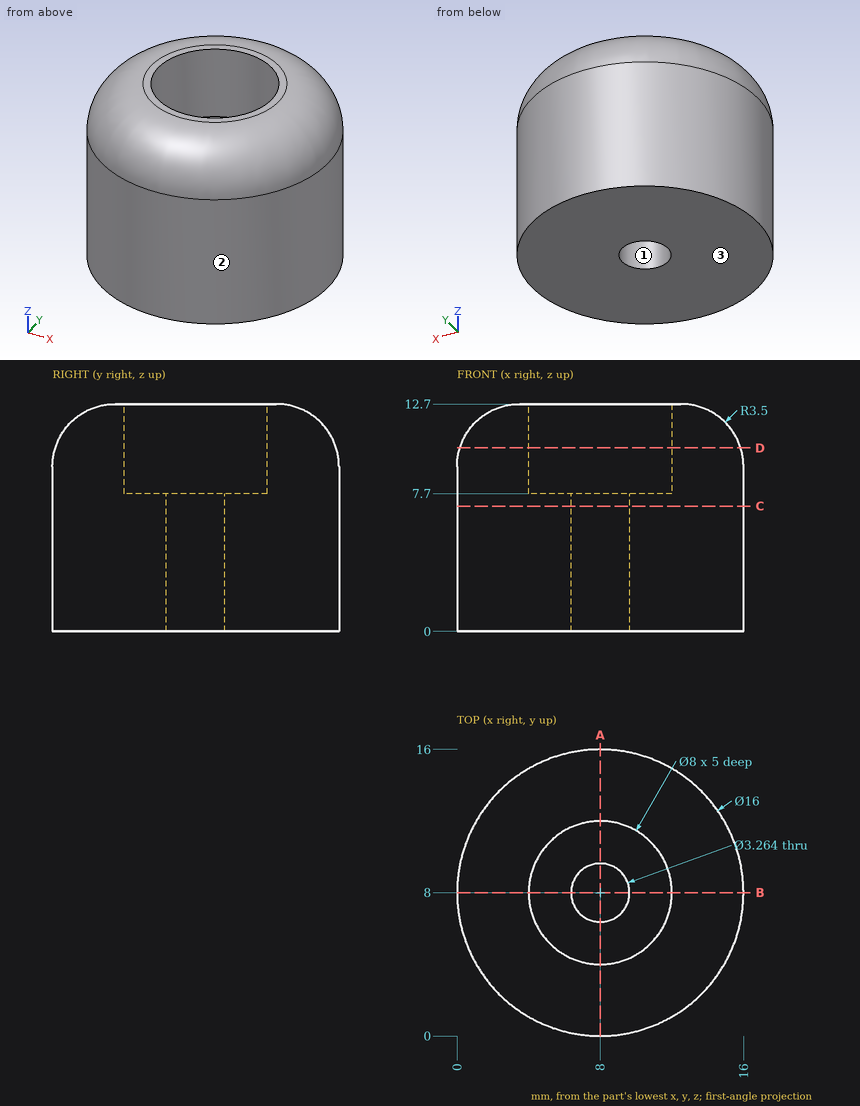
Verification items for this drawing (mm, ordinates from the low corner). Coordinates: 2 decimals unless noted, no trailing zeros. Write each loop counter-clockwise with the first axis right and the second up, starting at its lowest first coordinate (ties: lowest second). Pieces come first, ordered by that corner, then holes. Notation, with made-up numbers: (40, -40) -> (45, -40) arc R26 cw to (45, -16) -> close; hole circle Ø11 at (37, 0.25). An arc over 180 degrees is marked (long way). Use CSV: the item, a comma, the result in double quotes. Start each with the question number.
Item 1: Depth check by flat-ended pin: pin 1 Ø4 at (x, y) = (8, 8) entering from +Z; pin 2 Ø2 at (y, z) = (5, 3.5) entering from +X. Enter the tip coordinate at first touch or a pass-through.
Item 2: Cross-section at A-A, the plane x = 8. Record the cut outline in (y, z).
Item 3: Thickness scan on line 1 (Y direction, x = 8, z = 8.8); line 2 (Z direction, x = 7, y = 12.5); line 3 (Z direction, x = 4.5, y = 8.5). Record the ranges inside material, lowest first.
Item 4: Mould release check, pull along X, two halves, no side actions. Record for the marked faces 1, 2 and 3: released by +X, released by -X, zero draft, split by the parting line, or undercut.
Item 5: Cross-section at D-D, the plane z = 10.25. Record the cut outline in (x, y).
Item 6: Cross-section at C-C, the plane z = 7. Record the cut outline in (x, y), plus the area to 3 significant figures.
Answers:
1,pin 1,"z = 7.7"
1,pin 2,"x = 15.75"
2,outline,"(0, 0) -> (6.37, 0) -> (6.37, 7.7) -> (4, 7.7) -> (4, 12.7) -> (3.5, 12.7) arc R3.5 ccw to (0, 9.2) -> close; (9.63, 0) -> (16, 0) -> (16, 9.2) arc R3.5 ccw to (12.5, 12.7) -> (12, 12.7) -> (12, 7.7) -> (9.63, 7.7) -> close"
3,line 1,"0 to 4, 12 to 16"
3,line 2,"0 to 12.7"
3,line 3,"0 to 7.7"
4,face 1,"undercut"
4,face 2,"split by the parting line"
4,face 3,"zero draft"
5,outline,"circle Ø15.68 at (8, 8); hole circle Ø8 at (8, 8)"
6,outline,"circle Ø16 at (8, 8); hole circle Ø3.26 at (8, 8)"
6,area,"193 mm^2"
